Source: three-view drawing plus pictorial views. Frame: mm from the lowest corner of the part. Give positions to 0.01 mm unless a question says otherwise; leave off trailing zeros. Order: outer loops, then holes, each group sorted by start corner. A loop starts at its lowest first (then second) coordinate and runs counter-clockwise, first axis right, second up. Notation, with made-up numbers: (48.5, -26) -> (60.5, -26) arc R18 cw to (60.5, -6) -> close; hole circle Ø11 at (75, 32). An arc over 180 degrees is marked (long way). Answer in a Markdown table with one row per item. Add a question column.
Q1. Line query: line 1 along X through (y, z) = (0.75, 1.5). Output: solid intervals per line, ascending. Write a range as from..to.
Q2. Contact query for flat-ended pins moving along their axis: P1, Ø0.8, axis at y = 8, z = 1.5, coming from the +X side; P2, Ø0.9, axis at x = 53.5, z = 1, coming from the -Y side; P3, Ø1, axis at x = 45.5, z = 1, coming from the -Y side; P4, Ø0.6, axis at x = 1.5, z = 1, coming from the +Y side. Output: stop coordinate, or through.
Q3. Cut plane A-A on z = 1.15. Return the cut outline in (x, y).
Q4. Cut plane B-B on y = 1.5. Return the cut outline in (x, z), and give its area (3 significant figures).
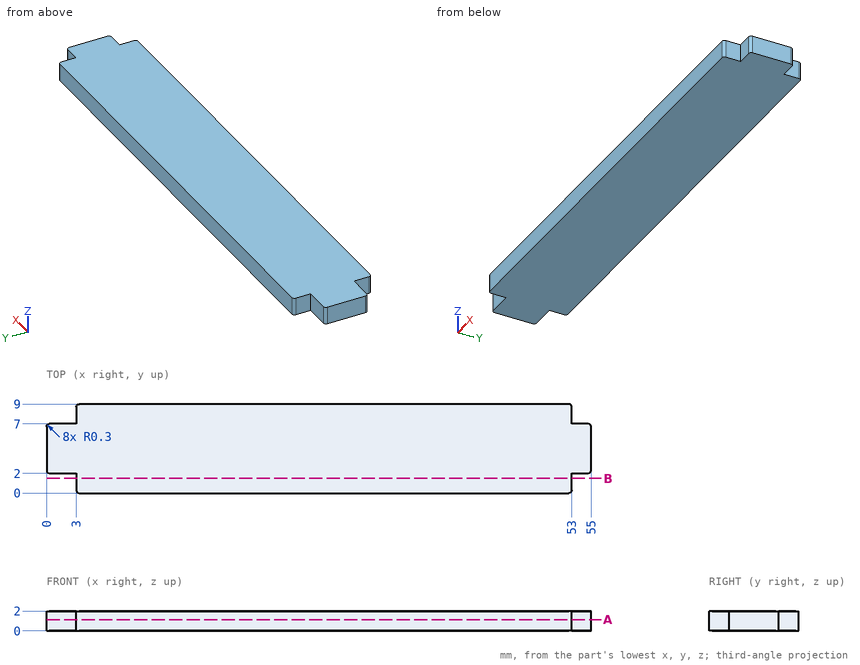
Completed:
| question | item | result |
|---|---|---|
| 1 | line 1 | x = 3..53 |
| 2 | P1 | stops at x = 53 |
| 2 | P2 | stops at y = 2 |
| 2 | P3 | stops at y = 0 |
| 2 | P4 | stops at y = 7 |
| 3 | outline | (0, 2.3) arc R0.3 ccw to (0.3, 2) -> (3, 2) -> (3, 0.3) arc R0.3 ccw to (3.3, 0) -> (52.7, 0) arc R0.3 ccw to (53, 0.3) -> (53, 2) -> (54.7, 2) arc R0.3 ccw to (55, 2.3) -> (55, 6.7) arc R0.3 ccw to (54.7, 7) -> (53, 7) -> (53, 8.7) arc R0.3 ccw to (52.7, 9) -> (3.3, 9) arc R0.3 ccw to (3, 8.7) -> (3, 7) -> (0.3, 7) arc R0.3 ccw to (0, 6.7) -> close |
| 4 | outline | (3, 0) -> (53, 0) -> (53, 2) -> (3, 2) -> close |
| 4 | area | 100 mm² |
